from build123d import *

# Parameters (mm, degrees)
BOSS_EXTRUDE1_DEPTH  = 3
M6_CLEARANCE_HOLE1_D = 6.6
CUT_EXTRUDE1_DEPTH   = 531.358070854


with BuildPart() as part:
    # Sketch1 → Boss-Extrude1 (new body)
    with BuildSketch(Plane.XY):
        with BuildLine():
            Line((-49.354733049, -25), (500.645266951, -25))
            Line((500.645266951, -25), (500.645266951, 175))
            Line((500.645266951, 175), (454.645266951, 175))
            ThreePointArc((454.645266951, 175), (453.231053388, 174.414213562), (452.645266951, 173))
            Line((452.645266951, 173), (452.645266951, 148))
            ThreePointArc((452.645266951, 148), (452.059480513, 146.585786438), (450.645266951, 146))
            Line((450.645266951, 146), (402.645266951, 146))
            ThreePointArc((402.645266951, 146), (401.231053388, 146.585786438), (400.645266951, 148))
            Line((400.645266951, 148), (400.645266951, 173))
            ThreePointArc((400.645266951, 173), (400.059480513, 174.414213562), (398.645266951, 175))
            Line((398.645266951, 175), (52.645266951, 175))
            ThreePointArc((52.645266951, 175), (51.231053388, 174.414213562), (50.645266951, 173))
            Line((50.645266951, 173), (50.645266951, 148))
            ThreePointArc((50.645266951, 148), (50.059480513, 146.585786438), (48.645266951, 146))
            Line((48.645266951, 146), (0.645266951, 146))
            ThreePointArc((0.645266951, 146), (-0.768946612, 146.585786438), (-1.354733049, 148))
            Line((-1.354733049, 148), (-1.354733049, 173))
            ThreePointArc((-1.354733049, 173), (-1.940519487, 174.414213562), (-3.354733049, 175))
            Line((-3.354733049, 175), (-49.354733049, 175))
            Line((-49.354733049, 175), (-49.354733049, -25))
        make_face()
    extrude(amount=BOSS_EXTRUDE1_DEPTH)

    # M6 Clearance Hole1 (through all)
    with Locations(Plane.XY.offset(3)):
        with Locations((225.645266951, -12.5), (225.645266951, 162.5), (488.145266951, -12.5), (488.145266951, 162.5), (-36.854733049, 162.5), (-36.854733049, -12.5)):
            Hole(M6_CLEARANCE_HOLE1_D / 2)

    # Sketch4 → Cut-Extrude1 (cut, through all)
    with BuildSketch(Plane.XY.offset(3)):
        with BuildLine():
            Line((-22.354733049, 6.35), (3.645266951, 6.35))
            ThreePointArc((3.645266951, 6.35), (5.059480513, 6.935786438), (5.645266951, 8.35))
            Line((5.645266951, 8.35), (5.645266951, 34.35))
            ThreePointArc((5.645266951, 34.35), (5.059480513, 35.764213562), (3.645266951, 36.35))
            Line((3.645266951, 36.35), (-22.354733049, 36.35))
            ThreePointArc((-22.354733049, 36.35), (-23.768946612, 35.764213562), (-24.354733049, 34.35))
            Line((-24.354733049, 34.35), (-24.354733049, 8.35))
            ThreePointArc((-24.354733049, 8.35), (-23.768946612, 6.935786438), (-22.354733049, 6.35))
        make_face()
    extrude(amount=-CUT_EXTRUDE1_DEPTH, mode=Mode.SUBTRACT)


solid = part.part
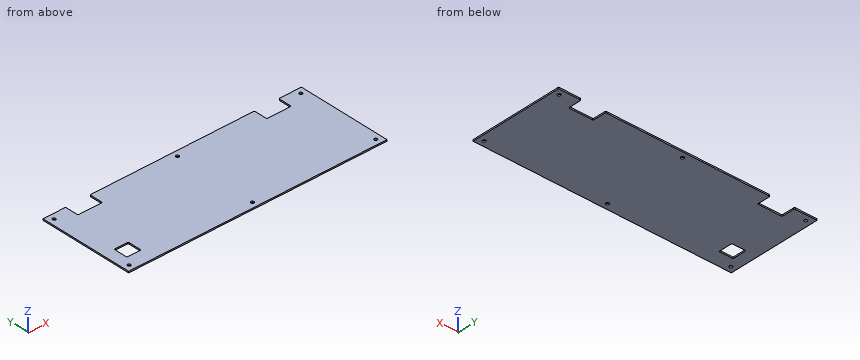
Model file for the job. Use its own axes, mm. Give positions to 0.01 mm unless a question says otherwise; leave off trailing zeros. Answer as CSV lines item,"result".
1. Band-saw the part on A-A (z = 2). Count the separate pieces of the cut face and the enclosed holes in it, and give its area (3 significant figures).
Responses:
separate pieces,"1"
enclosed holes,"7"
area,"106,000 mm2"
2. Pin check, flat tip, straight feed: pin 1 (1.5 mm diameter, centred on x = 425.5, z = 2, fed in from +Y). Stop position of the tip, or through.
Responses:
pin 1,"stops at y = 146"
3. Drill centre lines: L1, parallel to X at y = 162.5, z = 1.8; L2, parallel to X at y = 155, z = 0.9; L3, parallel to Y at x = -18, z = 1.9. Where is each one in solid material? Low to high. Write a range as [from, to].
Responses:
L1,"x = [-49.35, -40.15], [-33.55, -1.35], [50.65, 222.35], [228.95, 400.65], [452.65, 484.85], [491.45, 500.65]"
L2,"x = [-49.35, -1.35], [50.65, 400.65], [452.65, 500.65]"
L3,"y = [-25, 6.35], [36.35, 175]"
